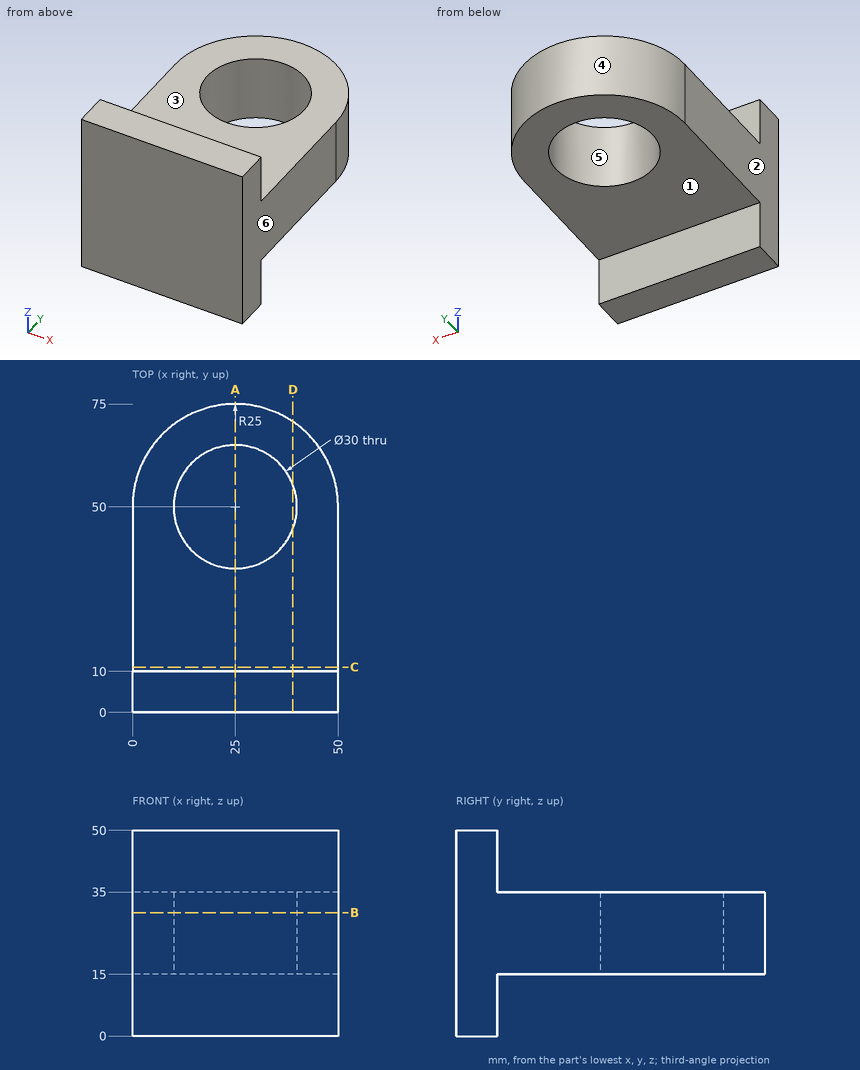
Answer from the drawing. Dimensions are ordinates in mm from the lowest x, y and z of the part. A direction names the side the tool comes from. Coordinates: 2 decimals unless noted, no trailing zeros. Write each loop counter-clockwise with the first axis right and the second up, starting at its lowest first coordinate (ties: lowest second). Pieces come first, ordered by that corner, then holes. Notation, with made-up numbers: M -12,-26 L 21,-26 A25 ccw 21,4 Z; hole C 46,57.5 d9. An arc over 180 degrees is marked long. Use one line per item in the form item = value. Start each with the question number.
1. Each of these flat-tipped pins is pushed along its axis until it touches: P1, Ø6, axis at x = 45, z = 16.5, coming from the +Y side; P2, Ø5, axis at x = 6.5, y = 49, coming from the +Z side; P3, Ø2, axis at x = 5, z = 42.5, coming from the +Y side. Where does it stop, or does it pass through?
2. The part is cut by section C-C (y = 11). Give the vertices of the cut face in (x, z), plus the area to 3 significant figures.
3. The part is cut by section B-B (z = 30). Give the vertices of the cut face in (x, y), plus the area to 3 significant figures.
4. The mould has two halves that part along Y. Classify the marked faces 4, 5 and 6: released by +Y, released by -Y, zero draft, split by the parting line, or undercut.
5. Straight lines are drawn through the part: probe 1 along Y at (x, z) = (25, 21); probe 2 along X at (y, z) = (49, 24); probe 3 along Z at (x, y) = (10, 52). For each, find the intervals that lie inside material, in ascending order. Write a range as from..to.
6. The part is cut by section A-A (x = 25). Give the vertices of the cut face in (y, z).
7. The part is cut by section D-D (x = 39). Give the vertices of the cut face in (y, z), plus the area to 3 significant figures.
8. A tool of negligible diameter and unlimited length cuts with its end or side. For the marked faces 1, 2 and 3, from which of +Z, -Z, +X, -X, +Y, -Y can it reach the whole face along a straight path? Write none if from no direction.
Evaluation:
q1.P1 = 68.33
q1.P2 = 35
q1.P3 = 10
q2.outline = M 0,15 L 50,15 L 50,35 L 0,35 Z
q2.area = 1,000 mm^2
q3.outline = M 0,0 L 50,0 L 50,50 A25 ccw 0,50 Z; hole C 25,50 d30
q3.area = 2,770 mm^2
q4.face_4 = released by +Y
q4.face_5 = undercut
q4.face_6 = zero draft
q5.probe_1 = 0..35, 65..75
q5.probe_2 = 0..10.03, 39.97..50
q5.probe_3 = 15..35
q6.outline = M 0,0 L 10,0 L 10,15 L 35,15 L 35,35 L 10,35 L 10,50 L 0,50 Z; M 65,15 L 75,15 L 75,35 L 65,35 Z
q7.outline = M 0,0 L 10,0 L 10,15 L 44.61,15 L 44.61,35 L 10,35 L 10,50 L 0,50 Z; M 55.39,15 L 70.71,15 L 70.71,35 L 55.39,35 Z
q7.area = 1,500 mm^2
q8.face_1 = -Z, +X, -X, +Y
q8.face_2 = +Z, -Z, -X, +Y, -Y
q8.face_3 = +Z, +X, -X, +Y
